```python
from build123d import *

# Parameters (mm, degrees)
SKETCH_1_W      = 80
SKETCH_1_H      = 10
SKETCH_1_R      = 1.25
SKETCH_1_R_2    = 1.7
EXTRUDE_1_DEPTH = 4
FILLET_1_R      = 3


with BuildPart() as part:
    # 草图1 → 凸台-拉伸1 (new body)
    with BuildSketch(Plane.XY):
        with Locations((40, 5)):
            Rectangle(SKETCH_1_W, SKETCH_1_H)
        with Locations((45, 5)):
            Circle(SKETCH_1_R, mode=Mode.SUBTRACT)
        with Locations((60, 5)):
            Circle(SKETCH_1_R, mode=Mode.SUBTRACT)
        with Locations((75, 5)):
            Circle(SKETCH_1_R, mode=Mode.SUBTRACT)
        with Locations((7.5, 5)):
            Circle(SKETCH_1_R_2, mode=Mode.SUBTRACT)
        with Locations((18.5, 5)):
            Circle(SKETCH_1_R_2, mode=Mode.SUBTRACT)
    extrude(amount=EXTRUDE_1_DEPTH)

    # 圆角1
    fillet_1_edges = [part.edges().sort_by_distance(p)[0] for p in [
        (0, 10, 2),
        (80, 10, 2),
        (80, 0, 2),
        (0, 0, 2),
    ]]
    fillet(fillet_1_edges, radius=FILLET_1_R)


solid = part.part
```
CAD build for the part. Positions are in the model's coordinates, mm. Coordinates: 2 decimals unless noted, no trailing zeros. Write each loop counter-clockwise with the first axis right and the second up, starting at its lowest first coordinate (ties: lowest second). Pieces come first, ordered by that corner, then holes. Notation, with made-up numbers: (82.25, 72) -> (91.25, 72) arc R27 cw to (91.25, 92) -> close; hole circle Ø6 at (89.25, 66). An arc over 180 degrees is marked (long way). Use CSV: the item, a comma, the result in double quotes. Start each with the question number.
Item 1: Band-saw the part on A-A, the plane x = 60. Write the cut outline in (y, z).
Item 2: Band-saw the part on B-B, the plane y = 5. Write the cut outline in (x, z).
Item 3: Drop flat-ended pins along their axis: P1, Ø1.5, axis at y = 2, z = 3.5, coming from the +X side; P2, Ø1.5, axis at y = 1.5, z = 2, coming from the -X side. Give the stop position or say it passes through.
Item 4: Band-saw the part on C-C, the plane z = 2.8. Write the cut outline in (x, y).
Item 5: Two-plate mould, pull along Y, no slides. Class faces 1 (the cylindrical face through (20.07, 4.35, 1.97)), 2 (the flat face through (39, 5, 4)), 3 (the cylindrical face through (0.86, 0.9, 2.03)): +Y half, -Y half, draft (parallel to the pull), parting line (faces both ways), or undercut.
Item 6: Wall check: probe 1 along Y at (x, z) = (60, 1.5); probe 2 along X at (y, z) = (4.5, 3.15); probe 3 along Y at (x, z) = (7.5, 1.95). Give the ranges that are in metal, low to high.
Item 7: Band-saw the part on D-D, the plane x = 7.5. Write the cut outline in (y, z), plus the area to 3 significant figures.
Response values:
1,outline,"(0, 0) -> (3.75, 0) -> (3.75, 4) -> (0, 4) -> close; (6.25, 0) -> (10, 0) -> (10, 4) -> (6.25, 4) -> close"
2,outline,"(0, 0) -> (5.8, 0) -> (5.8, 4) -> (0, 4) -> close; (9.2, 0) -> (16.8, 0) -> (16.8, 4) -> (9.2, 4) -> close; (20.2, 0) -> (43.75, 0) -> (43.75, 4) -> (20.2, 4) -> close; (46.25, 0) -> (58.75, 0) -> (58.75, 4) -> (46.25, 4) -> close; (61.25, 0) -> (73.75, 0) -> (73.75, 4) -> (61.25, 4) -> close; (76.25, 0) -> (80, 0) -> (80, 4) -> (76.25, 4) -> close"
3,P1,"stops at x = 79.99"
3,P2,"stops at x = 0.1"
4,outline,"(0, 3) arc R3 ccw to (3, 0) -> (77, 0) arc R3 ccw to (80, 3) -> (80, 7) arc R3 ccw to (77, 10) -> (3, 10) arc R3 ccw to (0, 7) -> close; hole circle Ø3.4 at (7.5, 5); hole circle Ø3.4 at (18.5, 5); hole circle Ø2.5 at (45, 5); hole circle Ø2.5 at (60, 5); hole circle Ø2.5 at (75, 5)"
5,face 1,"undercut"
5,face 2,"draft"
5,face 3,"-Y half"
6,probe 1,"y = 0 to 3.75, 6.25 to 10"
6,probe 2,"x = 0 to 5.88, 9.12 to 16.88, 20.12 to 43.85, 46.15 to 58.85, 61.15 to 73.85, 76.15 to 80"
6,probe 3,"y = 0 to 3.3, 6.7 to 10"
7,outline,"(0, 0) -> (3.3, 0) -> (3.3, 4) -> (0, 4) -> close; (6.7, 0) -> (10, 0) -> (10, 4) -> (6.7, 4) -> close"
7,area,"26.4 mm2"
